from build123d import *

# Parameters (mm, degrees)
BOSS_EXTRUDE1_DEPTH = 3
BOSS_EXTRUDE2_DEPTH = 21
SKETCH3_R           = 1.642484664
SKETCH3_R_2         = 1.292978033
CUT_EXTRUDE1_DEPTH  = 98.218880344


with BuildPart() as part:
    # Sketch1 → Boss-Extrude1 (new body)
    with BuildSketch(Plane.XY):
        Polygon((-82.599251445, -2.855918156), (-78.97237959, -6.297691035), (78.97237959, -6.297691035), (82.599251445, -2.855918156), (48.18152266, 33.412800394), (0, 46.774719198), (-48.18152266, 33.412800394), align=None)
    extrude(amount=BOSS_EXTRUDE1_DEPTH)

    # Sketch2 → Boss-Extrude2 (add)
    with BuildSketch(Plane.XY.offset(3)):
        Polygon((-44.808816074, 34.34813471), (-48.18152266, 33.412800394), (-50.590763675, 30.873990096), (-49.21255237, 29.566116402), (-48.352109151, 30.472834366), (-46.030911164, 28.270099723), (-46.891354383, 27.36338176), (-46.192513036, 26.700206083), (-44.440185395, 27.186169547), (-43.188437129, 28.505236993), (-43.445900356, 29.433619399), (-44.650438423, 29.099571429), (-45.505601226, 32.183188879), (-44.30106316, 32.517236849), align=None)
        Polygon((0, 46.774719198), (-3.372706586, 45.839384882), (-2.864953672, 44.008487021), (-1.660415605, 44.342534991), (-0.805252802, 41.25891754), (-2.009790868, 40.92486957), (-1.752327641, 39.996487164), (0, 39.5105237), (1.752327641, 39.996487164), (2.009790868, 40.92486957), (0.805252802, 41.25891754), (1.660415605, 44.342534991), (2.864953672, 44.008487021), (3.372706586, 45.839384882), align=None)
        Polygon((-78.811799125, -1.624981552), (-80.19001043, -0.317107858), (-82.599251445, -2.855918156), (-78.97237959, -6.297691035), (-76.215182645, -6.297691035), (-75.112389833, -5.135589888), (-76.490601138, -3.827716194), (-77.351044358, -4.734434158), (-79.672242345, -2.531699516), align=None)
        Polygon((48.18152266, 33.412800394), (44.808816074, 34.34813471), (44.30106316, 32.517236849), (45.505601226, 32.183188879), (44.650438423, 29.099571429), (43.445900356, 29.433619399), (43.188437129, 28.505236993), (44.440185395, 27.186169547), (46.192513036, 26.700206083), (46.891354383, 27.36338176), (46.030911164, 28.270099723), (48.352109151, 30.472834366), (49.21255237, 29.566116402), (50.590763675, 30.873990096), align=None)
        Polygon((75.112389833, -5.135589888), (76.215182645, -6.297691035), (78.97237959, -6.297691035), (82.599251445, -2.855918156), (80.19001043, -0.317107858), (78.811799125, -1.624981552), (79.672242345, -2.531699516), (77.351044358, -4.734434158), (76.490601138, -3.827716194), align=None)
    extrude(amount=BOSS_EXTRUDE2_DEPTH)

    # Sketch3 → Cut-Extrude1 (cut, through all)
    with BuildSketch(Plane.XY.offset(3)):
        with Locations((0, -2.554468846)):
            Circle(SKETCH3_R)
        with Locations((0, 15.270369354)):
            Circle(SKETCH3_R_2)
        with BuildLine():
            Line((-69.420990751, 3.767372692), (-50.828151114, 23.360137575))
            ThreePointArc((-50.828151114, 23.360137575), (-48.390560772, 24.283657942), (-46.150370534, 22.950884804))
            Line((-46.150370534, 22.950884804), (-33.182202355, 3.358119921))
            ThreePointArc((-33.182202355, 3.358119921), (-33.041187606, 0.282349963), (-35.683859821, -1.297691035))
            Line((-35.683859821, -1.297691035), (-67.244867638, -1.297691035))
            ThreePointArc((-67.244867638, -1.297691035), (-70.001241269, 0.518077396), (-69.420990751, 3.767372692))
        make_face()
        with BuildLine():
            Line((-25.543650537, 0.270832684), (-39.897767636, 26.707827652))
            ThreePointArc((-39.897767636, 26.707827652), (-40.022830858, 29.311497318), (-38.063031426, 31.030195292))
            Line((-38.063031426, 31.030195292), (-8.166425929, 39.321257781))
            ThreePointArc((-8.166425929, 39.321257781), (-5.611961803, 38.865088367), (-4.368822196, 36.58737429))
            Line((-4.368822196, 36.58737429), (-2.548801826, 1.859316834))
            ThreePointArc((-2.548801826, 1.859316834), (-3.368567317, -0.362754762), (-5.54469043, -1.297691035))
            Line((-5.54469043, -1.297691035), (-22.907199199, -1.297691035))
            ThreePointArc((-22.907199199, -1.297691035), (-24.441078457, -0.875910269), (-25.543650537, 0.270832684))
        make_face()
        with BuildLine():
            Line((5.54469043, -1.297691035), (22.907199199, -1.297691035))
            ThreePointArc((22.907199199, -1.297691035), (24.441078457, -0.875910269), (25.543650537, 0.270832684))
            Line((25.543650537, 0.270832684), (39.897767636, 26.707827652))
            ThreePointArc((39.897767636, 26.707827652), (40.022830858, 29.311497318), (38.063031426, 31.030195292))
            Line((38.063031426, 31.030195292), (8.166425929, 39.321257781))
            ThreePointArc((8.166425929, 39.321257781), (5.611961803, 38.865088367), (4.368822196, 36.58737429))
            Line((4.368822196, 36.58737429), (2.548801826, 1.859316834))
            ThreePointArc((2.548801826, 1.859316834), (3.368567317, -0.362754762), (5.54469043, -1.297691035))
        make_face()
        with BuildLine():
            Line((35.683859821, -1.297691035), (67.244867638, -1.297691035))
            ThreePointArc((67.244867638, -1.297691035), (70.001241269, 0.518077396), (69.420990751, 3.767372692))
            Line((69.420990751, 3.767372692), (50.828151114, 23.360137575))
            ThreePointArc((50.828151114, 23.360137575), (48.390560772, 24.283657942), (46.150370534, 22.950884804))
            Line((46.150370534, 22.950884804), (33.182202355, 3.358119921))
            ThreePointArc((33.182202355, 3.358119921), (33.041187606, 0.282349963), (35.683859821, -1.297691035))
        make_face()
    extrude(amount=-CUT_EXTRUDE1_DEPTH, mode=Mode.SUBTRACT)


solid = part.part
Could you check a few things on this model? Use its own coordinates, in mm. A direction names the side the tool comes from. Coordinates: 2 decimals unless noted, no trailing zeros. Order: outer loops, then holes, each group sorted by start corner. A loop starts at its lowest first (then second) coordinate and runs counter-clockwise, first axis right, second up. Notation, with made-up numbers: (77, -19.75) -> (116, -19.75) arc R13 ccw to (116, -15.75) -> close; hole circle Ø9 at (21, 0.5). An arc over 180 degrees is marked (long way). One line per question, with ' | ' between items.
Q1. On a 3-axis mill with a long thin cutter (end or side, diameter ignored), from which of +Z, -Z, +X, -X, +Y, -Y can I reach the whole of each face in a straight line? I mean faces 3 (the face through (-18, -6.298, 2)), 4 (the face through (24.4, -0.9, 1.5)), 5 (the face through (45.084, 30.663, 13.353)). Say none if no direction works.
Return value:
face 3: +Z, -Z, +X, -X, -Y | face 4: +Z, -Z | face 5: +Z
Q2. If I drill on L1, parallel to Y at x = 0, z = 1.25; L2, parallel to X at y = 32, z = 6.25; L3, parallel to Z at x = 6.5, y = 43, over which ranges is the centre line in solid material (lowest first)?
Return value:
L1: -6.3 to -4.2, -0.91 to 13.98, 16.56 to 46.77 | L2: -49.52 to -45.45, 45.45 to 49.52 | L3: 0 to 3
Q3. Imagine slicing it at B-B on x = -57.5. Please give me the cut outline in (y, z), and give its area (3 significant figures).
Return value:
outline: (-6.3, 0) -> (-1.3, 0) -> (-1.3, 3) -> (-6.3, 3) -> close; (16.33, 0) -> (23.59, 0) -> (23.59, 3) -> (16.33, 3) -> close | area: 36.8 mm²
Q4. Imagine slicing it at A-A on y = 20.5. Please give me the cut outline in (x, z), and give its area (3 significant figures).
Return value:
outline: (-60.44, 0) -> (-53.54, 0) -> (-53.54, 3) -> (-60.44, 3) -> close; (-44.53, 0) -> (-36.53, 0) -> (-36.53, 3) -> (-44.53, 3) -> close; (-3.53, 0) -> (3.53, 0) -> (3.53, 3) -> (-3.53, 3) -> close; (36.53, 0) -> (44.53, 0) -> (44.53, 3) -> (36.53, 3) -> close; (53.54, 0) -> (60.44, 0) -> (60.44, 3) -> (53.54, 3) -> close | area: 111 mm²
Q5. I'm going to push flat-ended pins straight in: P1, Ø2.5, axis at x = -13.5, z = 2, coming from the +Y side; P2, Ø0.9, axis at x = 59.5, z = 1.5, coming from the +Y side; P3, Ø2.5, axis at x = 17, z = 1, coming from the +Y side; P4, Ø2.5, axis at x = 0, y = -2.55, coming from the -Z side. Where does each tip first touch, or does it pass through?
Return value:
P1: y = 43.38 | P2: y = 21.96 | P3: y = 42.41 | P4: through
Q6. Imagine slicing it at C-C on z = 5. State how many separate pieces and enclosed holes the cut face has, and give its area (3 significant figures).
Return value:
separate pieces: 5 | enclosed holes: 0 | area: 115 mm²
Q7. Thinking about a two-plate mould opening in X: for faces 1 (the face through (-79, -4, 24)), 2 (the face through (40.037, 29.277, 1.521)), which applies, pulls with the +X half, pulls with the -X half, needs draft (parallel to the pull), parting line crosses it, or undercut?
Return value:
face 1: needs draft | face 2: undercut
Q8. Imagine slicing it at D-D on x = 13.5. Please give me the cut outline in (y, z).
Return value:
outline: (-6.3, 0) -> (-1.3, 0) -> (-1.3, 3) -> (-6.3, 3) -> close; (37.84, 0) -> (43.03, 0) -> (43.03, 3) -> (37.84, 3) -> close
